from build123d import *

# Parameters (mm, degrees)
F0_W     = 2
F0_H     = 25
F1_DEPTH = 10
F2_R     = 9.99999
F4_D     = 6
F6_D     = 3
F8_D     = 8


# Not quite as in the source:
# - a fillet or chamfer is up to 0.001 mm smaller than in the source, because OpenCascade refuses the exact size


with BuildPart() as f1:
    # F0 (on Top) → F1 (new body, symmetric)
    with BuildSketch(Plane.XY):
        with Locations((-21, -1)):
            Rectangle(F0_W, F0_H)
        Polygon((-22, 13.5), (-22, 11.5), (-20, 11.5), (20, 11.5), (22, 11.5), (22, 13.5), align=None)
        with Locations((21, -1)):
            Rectangle(F0_W, F0_H)
    extrude(amount=F1_DEPTH, both=True)

    # F2 (radius 10 in the source; OpenCascade refuses exactly that, so slightly less here)
    f2_edges = [f1.edges().sort_by_distance(p)[0] for p in [
        (21, -13.5, 10),
        (21, -13.5, -10),
    ]]
    fillet(f2_edges, radius=F2_R)

    # F4 (through all)
    with Locations(Plane(origin=(0, 13.5, 0), x_dir=(-1, 0, 0), z_dir=(0, 1, 0))):
        with Locations((0, 0)):
            Hole(F4_D / 2)

    # F6 (through all)
    with Locations(Plane(origin=(0, 13.5, 0), x_dir=(-1, 0, 0), z_dir=(0, 1, 0))):
        with Locations((-5, 5), (5, 5), (5, -5), (-5, -5)):
            Hole(F6_D / 2)

    # F8 (through all)
    with Locations(Plane.YZ.offset(22)):
        with Locations((-3.5, 0)):
            Hole(F8_D / 2)


solid = f1.part
The model under review builds one solid part; all positions refer to its coordinate system, in mm. A direction names the side the tool comes from. Round coordinates to 2 decimals unless told otherwise and drop trailing zeros. Write each loop counter-clockwise with the first axis right and the second up, starting at its lowest first coordinate (ties: lowest second). Pieces come first, ordered by that corner, then holes. Notation, with made-up numbers: M -17.5,53.25 L 18.5,53.25 A18 ccw 18.5,62.25 Z; hole C 70.25,-29.5 d11. An arc over 180 degrees is marked long. Use a Markdown table: item, result. Add a question column.
Q1. Machinability: for faces 5 (the face through (-6.2, 12.5, 4.1)), 6 (the face through (-3, 12, 10)), 7 (the face through (21.01, -10.65, 6.99)), 8 (the face through (20, 2, 0)), 9 (the face through (21.01, -10.65, -6.99)), which of the approach directions +Z, -Z, +X, -X, +Y, -Y give a long, thin tool a straight path to every point of the face, cutting with its end or side? Answer none if there is none.
Q2. We need section A-A, the plane x = 5. State the section outline as (y, z) points, plus the area to 3 significant figures.
Q3. The part is to be moulded in two halves that separate along Y. For faces 1 (the face through (-21.014, -2.633, -3.905)), 2 (the face through (-20, 2, 0)), 3 (the face through (-21, -13.5, 0)), 4 (the face through (0, 13.5, 5)), say which applies: pulls with the +Y half, pulls with the -Y half, needs draft (parallel to the pull), parting line crosses it, or undercut.
Q4. Insertion check: pin 1 (2.5 mm diameter, centred on x = -5, z = 5, fed in from -Y); pin 2 (6 mm diameter, centred on x = 1.5, z = -2.5, fed in from -Y); pin 3 (9 mm diameter, centred on y = -3.5, z = 0, fed in from +X). Each pin has a flat end and moves straight along its axis. Give the tip position at first contact, or say it passes through.
Q5. We need section C-C, the plane y = 10.75. State the section outline as (x, z) points, plus the area to 3 significant figures.
Q6. To check wall thickness, follow line 1 (Z direction, x = -5, y = 12.75); line 2 (X direction, y = -9.25, z = 1); line 3 (Z direction, x = 0, y = 12.3). State the ranges of each line that lie inside material, in increasing order.
Q7. We need section D-D, the plane z = 0.5. State the section outline as (x, y) points.
Q8. We need section B-B, the plane x = 0. State the section outline as (y, z) points.
Findings below:
| question | item | result |
|---|---|---|
| 1 | face 5 | +Y, -Y |
| 1 | face 6 | +Z, +X, -X, +Y, -Y |
| 1 | face 7 | +Z, +X, -Y |
| 1 | face 8 | +Z, -Z, -Y |
| 1 | face 9 | -Z, +X, -Y |
| 2 | outline | M 11.5,-10 L 13.5,-10 L 13.5,-6.5 L 11.5,-6.5 Z; M 11.5,-3.5 L 13.5,-3.5 L 13.5,3.5 L 11.5,3.5 Z; M 11.5,6.5 L 13.5,6.5 L 13.5,10 L 11.5,10 Z |
| 2 | area | 28.0 mm² |
| 3 | face 1 | undercut |
| 3 | face 2 | needs draft |
| 3 | face 3 | pulls with the -Y half |
| 3 | face 4 | pulls with the +Y half |
| 4 | pin 1 | passes through |
| 4 | pin 2 | stops at y = 11.5 |
| 4 | pin 3 | stops at x = 22 |
| 5 | outline | M -22,-10 L -20,-10 L -20,10 L -22,10 Z; M 20,-10 L 22,-10 L 22,10 L 20,10 Z |
| 5 | area | 80.0 mm² |
| 6 | line 1 | z = -10 to -6.5, -3.5 to 3.5, 6.5 to 10 |
| 6 | line 2 | x = -22 to -20, 20 to 22 |
| 6 | line 3 | z = -10 to -3, 3 to 10 |
| 7 | outline | M -22,-13.5 L -20,-13.5 L -20,-7.47 L -22,-7.47 Z; M -22,0.47 L -20,0.47 L -20,11.5 L -2.96,11.5 L -2.96,13.5 L -22,13.5 Z; M 2.96,11.5 L 20,11.5 L 20,0.47 L 22,0.47 L 22,13.5 L 2.96,13.5 Z; M 20,-13.49 L 22,-13.49 L 22,-7.47 L 20,-7.47 Z |
| 8 | outline | M 11.5,-10 L 13.5,-10 L 13.5,-3 L 11.5,-3 Z; M 11.5,3 L 13.5,3 L 13.5,10 L 11.5,10 Z |
